Geometry: final body of the model. Coordinates: model frame, mm. A direction names the side the tool comes from. Coordinates: 2 decimals unless noted, no trailing zeros.
from build123d import *

# Parameters (mm, degrees)
SKETCH2_W                      = 101.6
SKETCH2_H                      = 101.6
BOSS_EXTRUDE1_DEPTH            = 6.35
F_6_32_TAPPED_HOLE1_AT_2_COUNT = 2
F_6_32_TAPPED_HOLE1_AT_2_PITCH = 95.25


with BuildPart() as part:
    # Sketch2 → Boss-Extrude1 (new body)
    with BuildSketch(Plane.XY):
        with Locations((50.8, 50.8)):
            Rectangle(SKETCH2_W, SKETCH2_H)
    extrude(amount=BOSS_EXTRUDE1_DEPTH)

    # Sketch7 → #6-32 Tapped Hole1 (revolve, cut)
    with BuildSketch(Plane(origin=(3.175, 101.6, 3.175), x_dir=(0, 0, 1), z_dir=(1, 0, 0))):
        Polygon((0, 0), (0, 10.21069403), (1.35255, 9.398), (1.35255, 0), align=None)
    f_6_32_tapped_hole1 = revolve(axis=Axis((3.175, 107.95, 3.175), (0, -1, 0)), mode=Mode.SUBTRACT)

    # #6-32 Tapped Hole1 at 2: #6-32 Tapped Hole1 ×2
    with Locations(*[(i * F_6_32_TAPPED_HOLE1_AT_2_PITCH, 0, 0) for i in range(1, F_6_32_TAPPED_HOLE1_AT_2_COUNT)]):
        add(f_6_32_tapped_hole1, mode=Mode.SUBTRACT)

    # Mirror1: #6-32 Tapped Hole1 across plane
    add(f_6_32_tapped_hole1.mirror(Plane.ZX.offset(50.8)), mode=Mode.SUBTRACT)

    # Mirror1 copy 1 sketch → Mirror1 copy 1 (revolve, cut)
    with BuildSketch(Plane(origin=(98.425, 0, 3.175), x_dir=(0, 0, 1), z_dir=(1, 0, 0))):
        Polygon((0, 0), (0, -10.21069403), (1.35255, -9.398), (1.35255, 0), align=None)
    revolve(axis=Axis((98.425, -6.35, 3.175), (0, -1, 0)), mode=Mode.SUBTRACT)


solid = part.part
Item 1: Material intervals for probe 1 along X at (y, z) = (8, 3), sorted ascending.
Derived:
probe 1: x = 0 to 1.83, 4.52 to 97.08, 99.77 to 101.6
Item 2: Set-up query: faces 4 (the flat face through (50, 52, 0)), 5 (the cylindrical face through (99.745, 4.633, 2.882)), 6 (the cylindrical face through (3.998, 96.967, 2.102)). Return all of +Z, -Z, +X, -X, +Y, -Y with unobstructed straight access to the full face (end or side cutting, diameter ignored); none if empty.
Derived:
face 4: -Z, +X, -X, +Y, -Y
face 5: -Y
face 6: +Y
Item 3: Pull-direction query (Z, two-part tool) for faces 1 (the flat face through (50, 52, 6.35)), 2 (the flat face through (50, 0, 3)), 3 (the conical face through (98.23, 91.53, 3.3)); classes: released by +Z, released by -Z, zero draft, split by the parting line, or undercut.
Derived:
face 1: released by +Z
face 2: zero draft
face 3: undercut
Item 4: Pin query (flat end, axial travel): pin 1 (1.6 mm diameter, centred on x = 3.175, z = 3.175, fed in from +Y). Return the tip coordinate at first contact, or that it passes through.
Derived:
pin 1: stops at y = 91.87
